The model under review builds one solid part; all positions refer to its coordinate system, in mm. A direction names the side the tool comes from. Coordinates: 2 decimals unless noted, no trailing zeros. Write each loop counter-clockwise with the first axis right and the second up, starting at its lowest first coordinate (ties: lowest second). Pieces come first, ordered by that corner, then holes. Notation, with made-up numbers: M -22.5,61.5 L -2.5,61.5 A18 cw -2.5,66.5 Z; hole C -7,46.25 d3. An arc over 180 degrees is marked long. Answer as a JSON object with one key per item and string values.
```python
from build123d import *

# Parameters (mm, degrees)
CHAMFER_1_SIZE      = 1
CUT_EXTRUDE_1_REACH = 42
SKETCH_2_R          = 6
SKETCH_2_R_2        = 11.75
CUT_EXTRUDE_2_REACH = 42
SKETCH_3_R          = 11.5
SKETCH_4_R          = 17.5
CUT_EXTRUDE_3_DEPTH = 24


with BuildPart() as part:
    # 스케치1 → 회전1 (revolve)
    with BuildSketch(Plane.XY, mode=Mode.PRIVATE) as revolve_1_sk:
        Polygon((-150, 0), (-150, 30), (-97.5, 30), (-97.5, 38), (-40.15, 38), (-40.15, 40), (-35, 40), (-35, 5), (-43.5, 5), (-43.5, 0), align=None)
    revolve(revolve_1_sk.sketch.rotate(Axis((0, 0, 0), (0, 1, 0)), 270), axis=Axis((0, 0, 0), (0, 1, 0)))  # turned: the seam where the file's is

    # 모따기1
    chamfer_1_edges = [part.edges().sort_by_distance(p)[0] for p in [
        (0, 0, 43.5),
        (0, 5, 35),
    ]]
    chamfer(chamfer_1_edges, length=CHAMFER_1_SIZE)

    # 스케치2 → 컷-돌출1 (cut, up to next)
    with BuildSketch(Plane(origin=(0, 0, 0), x_dir=(1, 0, 0), z_dir=(0, 1, 0)), mode=Mode.PRIVATE) as cut_extrude_1_sk1:
        with Locations(Location((-60, 60, 0), (0, 0, 90))):  # turned: the seam where the file's is
            Circle(SKETCH_2_R)
    cut_extrude_1_tool1 = extrude(cut_extrude_1_sk1.sketch, amount=CUT_EXTRUDE_1_REACH, mode=Mode.PRIVATE) & part.part
    add(cut_extrude_1_tool1.solids().sort_by_distance((-60, 0, -60))[0], mode=Mode.SUBTRACT)
    # 스케치2 → 컷-돌출1 (cut, up to next)
    with BuildSketch(Plane(origin=(0, 0, 0), x_dir=(1, 0, 0), z_dir=(0, 1, 0)), mode=Mode.PRIVATE) as cut_extrude_1_sk2:
        with Locations(Location((-89.802561211, 89.802561211, 0), (0, 0, 90))):  # turned: the seam where the file's is
            Circle(SKETCH_2_R_2)
    cut_extrude_1_tool2 = extrude(cut_extrude_1_sk2.sketch, amount=CUT_EXTRUDE_1_REACH, mode=Mode.PRIVATE) & part.part
    add(cut_extrude_1_tool2.solids().sort_by_distance((-89.802561, 0, -89.802561))[0], mode=Mode.SUBTRACT)
    # 스케치2 → 컷-돌출1 (cut, up to next)
    with BuildSketch(Plane(origin=(0, 0, 0), x_dir=(1, 0, 0), z_dir=(0, 1, 0)), mode=Mode.PRIVATE) as cut_extrude_1_sk3:
        with Locations(Location((89.802561211, 89.802561211, 0), (0, 0, 90))):  # turned: the seam where the file's is
            Circle(SKETCH_2_R_2)
    cut_extrude_1_tool3 = extrude(cut_extrude_1_sk3.sketch, amount=CUT_EXTRUDE_1_REACH, mode=Mode.PRIVATE) & part.part
    add(cut_extrude_1_tool3.solids().sort_by_distance((89.802561, 0, -89.802561))[0], mode=Mode.SUBTRACT)
    # 스케치2 → 컷-돌출1 (cut, up to next)
    with BuildSketch(Plane(origin=(0, 0, 0), x_dir=(1, 0, 0), z_dir=(0, 1, 0)), mode=Mode.PRIVATE) as cut_extrude_1_sk4:
        with Locations(Location((89.802561211, -89.802561211, 0), (0, 0, 90))):  # turned: the seam where the file's is
            Circle(SKETCH_2_R_2)
    cut_extrude_1_tool4 = extrude(cut_extrude_1_sk4.sketch, amount=CUT_EXTRUDE_1_REACH, mode=Mode.PRIVATE) & part.part
    add(cut_extrude_1_tool4.solids().sort_by_distance((89.802561, 0, 89.802561))[0], mode=Mode.SUBTRACT)
    # 스케치2 → 컷-돌출1 (cut, up to next)
    with BuildSketch(Plane(origin=(0, 0, 0), x_dir=(1, 0, 0), z_dir=(0, 1, 0)), mode=Mode.PRIVATE) as cut_extrude_1_sk5:
        with Locations(Location((-89.802561211, -89.802561211, 0), (0, 0, 90))):  # turned: the seam where the file's is
            Circle(SKETCH_2_R_2)
    cut_extrude_1_tool5 = extrude(cut_extrude_1_sk5.sketch, amount=CUT_EXTRUDE_1_REACH, mode=Mode.PRIVATE) & part.part
    add(cut_extrude_1_tool5.solids().sort_by_distance((-89.802561, 0, 89.802561))[0], mode=Mode.SUBTRACT)

    # 스케치3 → 컷-돌출2 (cut, up to next)
    with BuildSketch(Plane(origin=(0, 0, 0), x_dir=(1, 0, 0), z_dir=(0, 1, 0)), mode=Mode.PRIVATE) as cut_extrude_2_sk1:
        with Locations(Location((-28.338059011, 69.440293861, 0), (0, 0, 90))):  # turned: the seam where the file's is
            Circle(SKETCH_3_R)
    cut_extrude_2_tool1 = extrude(cut_extrude_2_sk1.sketch, amount=CUT_EXTRUDE_2_REACH, mode=Mode.PRIVATE) & part.part
    add(cut_extrude_2_tool1.solids().sort_by_distance((-28.338059, 0, -69.440294))[0], mode=Mode.SUBTRACT)
    # 스케치3 → 컷-돌출2 (cut, up to next)
    with BuildSketch(Plane(origin=(0, 0, 0), x_dir=(1, 0, 0), z_dir=(0, 1, 0)), mode=Mode.PRIVATE) as cut_extrude_2_sk2:
        with Locations(Location((69.440293861, 28.338059011, 0), (0, 0, 90))):  # turned: the seam where the file's is
            Circle(SKETCH_3_R)
    cut_extrude_2_tool2 = extrude(cut_extrude_2_sk2.sketch, amount=CUT_EXTRUDE_2_REACH, mode=Mode.PRIVATE) & part.part
    add(cut_extrude_2_tool2.solids().sort_by_distance((69.440294, 0, -28.338059))[0], mode=Mode.SUBTRACT)
    # 스케치3 → 컷-돌출2 (cut, up to next)
    with BuildSketch(Plane(origin=(0, 0, 0), x_dir=(1, 0, 0), z_dir=(0, 1, 0)), mode=Mode.PRIVATE) as cut_extrude_2_sk3:
        with Locations(Location((28.338059011, -69.440293861, 0), (0, 0, 90))):  # turned: the seam where the file's is
            Circle(SKETCH_3_R)
    cut_extrude_2_tool3 = extrude(cut_extrude_2_sk3.sketch, amount=CUT_EXTRUDE_2_REACH, mode=Mode.PRIVATE) & part.part
    add(cut_extrude_2_tool3.solids().sort_by_distance((28.338059, 0, 69.440294))[0], mode=Mode.SUBTRACT)
    # 스케치3 → 컷-돌출2 (cut, up to next)
    with BuildSketch(Plane(origin=(0, 0, 0), x_dir=(1, 0, 0), z_dir=(0, 1, 0)), mode=Mode.PRIVATE) as cut_extrude_2_sk4:
        with Locations(Location((-69.440293861, -28.338059011, 0), (0, 0, 90))):  # turned: the seam where the file's is
            Circle(SKETCH_3_R)
    cut_extrude_2_tool4 = extrude(cut_extrude_2_sk4.sketch, amount=CUT_EXTRUDE_2_REACH, mode=Mode.PRIVATE) & part.part
    add(cut_extrude_2_tool4.solids().sort_by_distance((-69.440294, 0, 28.338059))[0], mode=Mode.SUBTRACT)

    # 스케치4 → 컷-돌출3 (cut)
    with BuildSketch(Plane(origin=(0, 0, 0), x_dir=(1, 0, 0), z_dir=(0, 1, 0))):
        with Locations(Location((-28.338059011, 69.440293861, 0), (0, 0, 270))):  # turned: the seam where the file's is
            Circle(SKETCH_4_R)
        with Locations(Location((-69.440293861, -28.338059011, 0), (0, 0, 270))):  # turned: the seam where the file's is
            Circle(SKETCH_4_R)
        with Locations(Location((69.440293861, 28.338059011, 0), (0, 0, 270))):  # turned: the seam where the file's is
            Circle(SKETCH_4_R)
        with Locations(Location((28.338059011, -69.440293861, 0), (0, 0, 270))):  # turned: the seam where the file's is
            Circle(SKETCH_4_R)
    extrude(amount=CUT_EXTRUDE_3_DEPTH, mode=Mode.SUBTRACT)


solid = part.part
```
(1) Wall thickness on line 1 along X through (y, z) = (2.5, 100.5); line 2 along X through (y, z) = (37, -59); line 3 along Z through (x, y) = (-83.5, 20.5): over which ranges is each line inside the solid? List them lowest first. Write a range as from..to.
Results list:
{"line 1": "-111.35..-94.66, -84.94..84.94, 94.66..111.35", "line 2": "-77.62..-65.92, -54.08..-33.16, -23.52..77.62", "line 3": "-124.61..-99.72, -79.89..17.92, 38.76..79.89, 99.72..124.61"}
(2) For pin 1 Ø17.5 at (x, z) = (-61.5, 27.5) entering from -Y; pin 2 Ø3 at (x, z) = (-85.5, -27) entering from +Y; pin 3 Ø1 at (x, y) = (-116, 24) entering from +Z, all flat-tipped, find the tip position at first contact; note any pin that passes through.
Results list:
{"pin 1": "y = 24", "pin 2": "y = 38", "pin 3": "z = 95.71"}
(3) Draft analysis for pull direction Z (two halves, no side actions). For faces 4 (the face through (31, 0, -35)), 5 (the face through (17, 24, 73)), 6 (the face through (91.273, 15.21, 119.035)), state which applies: released by +Z, released by -Z, zero draft, split by the parting line, or undercut.
Results list:
{"face 4": "zero draft", "face 5": "undercut", "face 6": "split by the parting line"}
(4) For faces 1 (the face through (-2, 30, -98)), 2 (the face through (53.915, 11.832, -20.263)), 3 (the face through (58.04, 30.9, -26.84)), list the 3-axis set-ups (+Z, -Z, +X, -X, +Y, -Y) from which the entire face can be reached by the end or side of a thin tool; tool diameter is ignored.
Results list:
{"face 1": "+Y", "face 2": "-Y", "face 3": "+Y, -Y"}
(5) Add section A-A on x = 0. Give the boundary of the cut face in (y, z).
Results list:
{"outline": "M 0,-150 L 30,-150 L 30,-97.5 L 38,-97.5 L 38,-40.15 L 40,-40.15 L 40,-35 L 6,-35 L 5,-36 L 5,-43.5 L 1,-43.5 L 0,-44.5 Z; M 0,44.5 L 1,43.5 L 5,43.5 L 5,36 L 6,35 L 40,35 L 40,40.15 L 38,40.15 L 38,97.5 L 30,97.5 L 30,150 L 0,150 Z"}
(6) Add section B-B on z = 0. Give the boundary of the cut face in (x, y), and give its area (3 significant figures).
Results list:
{"outline": "M -150,0 L -44.5,0 L -43.5,1 L -43.5,5 L -36,5 L -35,6 L -35,40 L -40.15,40 L -40.15,38 L -97.5,38 L -97.5,30 L -150,30 Z; M 35,6 L 36,5 L 43.5,5 L 43.5,1 L 44.5,0 L 150,0 L 150,30 L 97.5,30 L 97.5,38 L 40.15,38 L 40.15,40 L 35,40 Z", "area": "7,830 mm²"}
(7) Add section C-C on z = -126.5. Give the boundary of the cut face in (x, y), and give its area (3 significant figures).
Results list:
{"outline": "M -80.61,0 L 80.61,0 L 80.61,30 L -80.61,30 Z", "area": "4,840 mm²"}
